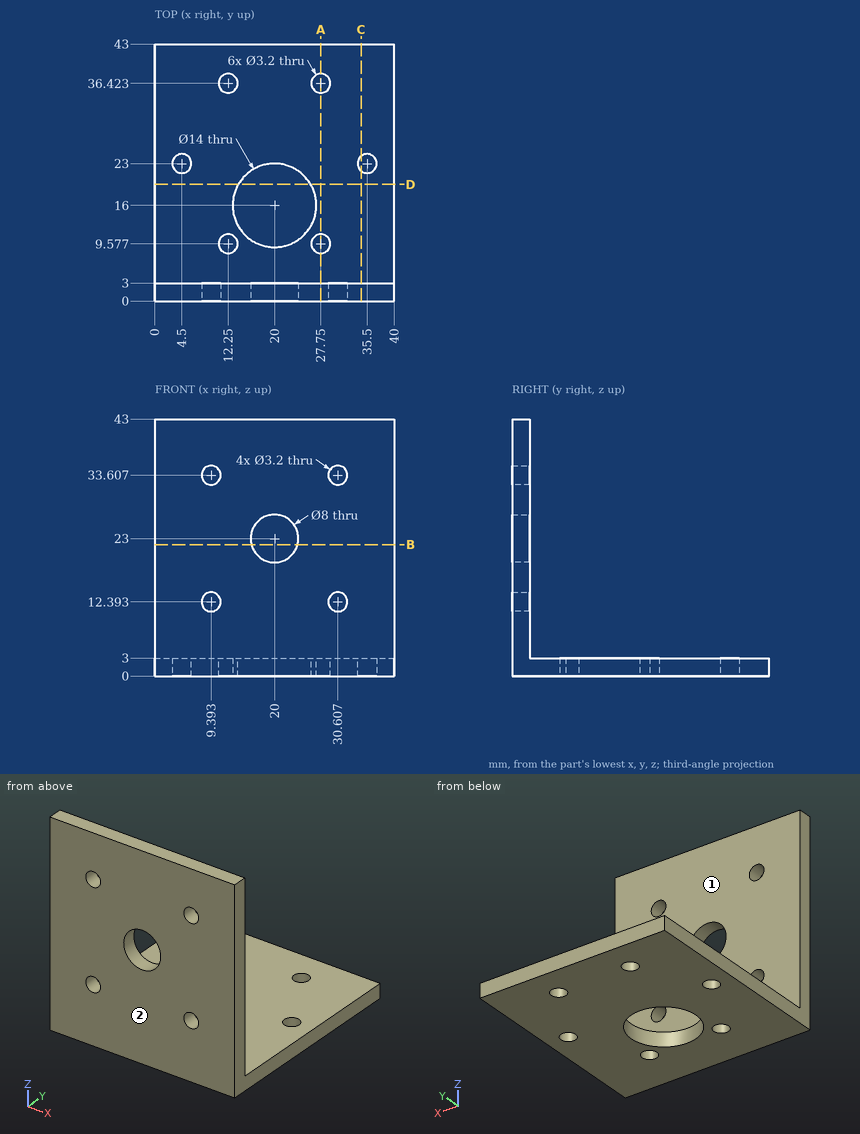
Could you check a few things on this drawing? It's one solid part, dimensions in mm from its lowest x, y, z. A direction names the side the tool comes from. Round coordinates to 2 decimals unless told otherwise and drop trailing zeros. Write each loop counter-clockwise with the first axis right and the second up, starting at its lowest first coordinate (ties: lowest second). Pieces come first, ordered by that corner, then holes. Notation, with made-up numbers: (74, 76.5) -> (82, 76.5) arc R20 ccw to (82, 97.5) -> close; hole circle Ø7 at (77.25, -23). An arc over 180 degrees is marked (long way). Use a Markdown table: item, result.
1. If we section it at A-A (x = 27.75): List the corners of the cut face in (y, z) for me.
Answer key:
| item | result |
|---|---|
| outline | (0, 0) -> (7.98, 0) -> (7.98, 3) -> (3, 3) -> (3, 43) -> (0, 43) -> close; (11.18, 0) -> (34.82, 0) -> (34.82, 3) -> (11.18, 3) -> close; (38.02, 0) -> (43, 0) -> (43, 3) -> (38.02, 3) -> close |
2. If we section it at D-D (y = 19.5): List the corners of the cut face in (x, z) for me.
Answer key:
| item | result |
|---|---|
| outline | (0, 0) -> (13.94, 0) -> (13.94, 3) -> (0, 3) -> close; (26.06, 0) -> (40, 0) -> (40, 3) -> (26.06, 3) -> close |
3. If we section it at B-B (z = 22): List the corners of the cut face in (x, y) for me.
Answer key:
| item | result |
|---|---|
| outline | (0, 0) -> (16.13, 0) -> (16.13, 3) -> (0, 3) -> close; (23.87, 0) -> (40, 0) -> (40, 3) -> (23.87, 3) -> close |
4. Please list where these lines run through material, in increasing order: probe 1 along Y at (x, z) = (27.75, 1.6); probe 2 along Y at (x, z) = (9.5, 29).
Answer key:
| item | result |
|---|---|
| probe 1 | y = 0 to 7.98, 11.18 to 34.82, 38.02 to 43 |
| probe 2 | y = 0 to 3 |
5. If we section it at C-C (x = 34.5): List the corners of the cut face in (y, z) for me.
Answer key:
| item | result |
|---|---|
| outline | (0, 0) -> (21.75, 0) -> (21.75, 3) -> (3, 3) -> (3, 43) -> (0, 43) -> close; (24.25, 0) -> (43, 0) -> (43, 3) -> (24.25, 3) -> close |
6. Which directions (+Z, -Z, +X, -X, +Y, -Y) give clear straight access to the entire face, cutting with the end or side of a thin tool? Please do the marked faces 1 and 2.
Answer key:
| item | result |
|---|---|
| face 1 | +Z, +X, -X, +Y |
| face 2 | +Z, -Z, +X, -X, -Y |
7. For pin 1 Ø4 at (x, z) = (9.39, 12.39) entering from -Y; pin 2 Ø4 at (x, y) = (12.25, 9.58) entering from +Z; pin 3 Ø3.5 at (x, z) = (9.39, 33.61) entering from +Y, each with a flat end and sliding along its axis, tell me the tip position at first contact or that it passes through.
Answer key:
| item | result |
|---|---|
| pin 1 | stops at y = 0 |
| pin 2 | stops at z = 3 |
| pin 3 | stops at y = 3 |
